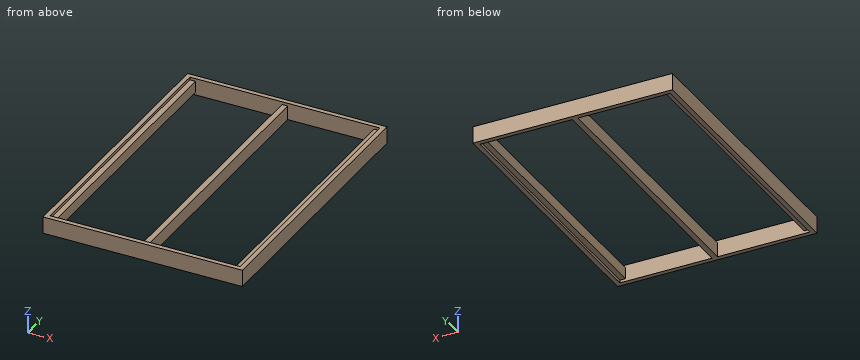
from build123d import *

# Parameters (mm, degrees)
F0_W     = 1352.55
F0_H     = 1889.125
F0_W_2   = 1289.05
F0_H_2   = 1825.625
F1_DEPTH = 114.3
F2_W     = 1825.625
F2_H     = 76.2
F3_DEPTH = 38.1
F4_W     = 1825.625
F4_H     = 76.2
F5_DEPTH = 38.1
F6_W     = 38.1
F6_H     = 95.25
F7_DEPTH = 1825.625


with BuildPart() as f1:
    # F0 (on Top) → F1 (new body)
    with BuildSketch(Plane.XY):
        Rectangle(F0_W, F0_H)
        Rectangle(F0_W_2, F0_H_2, mode=Mode.SUBTRACT)
    extrude(amount=F1_DEPTH)

    # F2 (on face) → F3 (join)
    with BuildSketch(Plane(origin=(644.525, 0, 0), x_dir=(0, -1, 0), z_dir=(-1, 0, 0))):
        with Locations((0, 57.15)):
            Rectangle(F2_W, F2_H)
    extrude(amount=F3_DEPTH)

    # F4 (on face) → F5 (join)
    with BuildSketch(Plane.YZ.offset(-644.525)):
        with Locations((0, 57.15)):
            Rectangle(F4_W, F4_H)
    extrude(amount=F5_DEPTH)

    # F6 (on face) → F7 (join, through all)
    with BuildSketch(Plane.XZ.offset(-912.8125)):
        with Locations((0, 47.625)):
            Rectangle(F6_W, F6_H)
    extrude(amount=F7_DEPTH)


solid = f1.part
For this review, take the finished solid that the model builds, in its own axes (mm). Give positions to 0.01 mm unless a question says otherwise; leave off trailing zeros. Loops run counter-clockwise (first coordinate to the right, second up) from the corner with the lowest first, then second, coordinate; pieces in that order, holes last. Notation, with made-up numbers: (19.25, 8.5) - (49.25, 8.5) arc R14 ccw to (49.25, 22.5) - close; hole circle Ø4 at (-2, -18). An arc over 180 degrees is marked (long way). Write each question's results on one line, items separated by ' | '.
(1) Take a section at B-B (y = 0). Give the boundary of the cut face in (x, z) (3 decimals), then the cut area to 3 significant figures.
Conclusion:
outline: (-676.275, 0) - (-644.525, 0) - (-644.525, 19.05) - (-606.425, 19.05) - (-606.425, 95.25) - (-644.525, 95.25) - (-644.525, 114.3) - (-676.275, 114.3) - close; (-19.05, 0) - (19.05, 0) - (19.05, 95.25) - (-19.05, 95.25) - close; (606.425, 19.05) - (644.525, 19.05) - (644.525, 0) - (676.275, 0) - (676.275, 114.3) - (644.525, 114.3) - (644.525, 95.25) - (606.425, 95.25) - close | area: 16,700 mm^2
(2) Take a section at C-C (x = 483). Give the boundary of the cut face in (y, z).
Conclusion:
outline: (-944.56, 0) - (-912.81, 0) - (-912.81, 114.3) - (-944.56, 114.3) - close; (912.81, 0) - (944.56, 0) - (944.56, 114.3) - (912.81, 114.3) - close
(3) Take a section at A-A (z = 39). State how many separate pieces and enclosed holes the cut face has, then the cut area to 3 significant figures.
Conclusion:
separate pieces: 1 | enclosed holes: 2 | area: 410,000 mm^2
(4) For pin 1 Ø19 at (x, y) = (-627, -97.5) entering from -Z, flat-tipped, find the tip position at first contact; note if it passes through.
Conclusion:
pin 1: z = 19.05
(5) For line 1 along X through (y, z) = (256.5, 80) (3 decimals); line 2 along X through (y, z) = (-100, 7) (3 decimals); line 3 along Y through (x, z) = (246, 17.5), list the stretches that pass through material, from the lowest coordinate up.
Conclusion:
line 1: -676.275 to -606.425, -19.05 to 19.05, 606.425 to 676.275 | line 2: -676.275 to -644.525, -19.05 to 19.05, 644.525 to 676.275 | line 3: -944.56 to -912.81, 912.81 to 944.56
